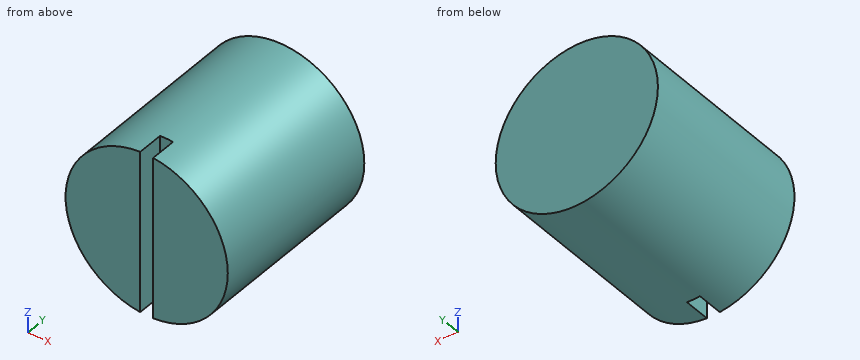
Autodesk Fusion 360 part; units mm, degrees
sketch "Sketch1" plane through (0, 0, 0) normal (0, 1, 0) x (1, 0, 0)
  circle A0 centre (0, 0) radius 5
  dimension "d1" = 10
extrude "Extrude1" add sketch "Sketch1" along normal blind 11
sketch "Sketch2" plane through (0, 0, 0) normal (1, 0, 0) x (0, 1, 0)
sketch "Sketch3" plane through (0, 0, 0) normal (0, 1, 0) x (1, 0, 0)
  circle A0 centre (0, 0) radius 5
  line L0 (-0.398, -4.9841) -> (-0.398, 4.9841)
  line L1 (0.398, 4.9841) -> (0.398, -4.9841)
  line L2 (-0.398, -4.9841) -> (-0.398, -5.1)
  line L3 (-0.398, -5.1) -> (0.4, -5.1)
  line L4 (0.4, -5.1) -> (0.398, -4.9841)
  line L5 (0.398, 4.9841) -> (0.398, 5.2684)
  line L6 (0.398, 5.2684) -> (-0.5, 5.2684)
  line L7 (-0.5, 5.2684) -> (-0.398, 4.9841)
extrude "Extrude2" cut sketch "Sketch3" along normal blind 1.6 contours A0 L0 L1 | A0 L5 L6 L7 | A0 L2 L3 L4
CAD build for the part. Positions are in the model's coordinates, mm. Give positions to 0.01 mm unless a question says otherwise; leave off trailing zeros. Order: outer loops, then holes, each group sorted by start corner. A loop starts at its lowest first (then second) coordinate and runs counter-clockwise, first axis right, second up. Notation, with made-up numbers: (-15, 13.5) - (4, 13.5) arc R4 ccw to (4, 17.5) - close; hole circle Ø11 at (37, -23.5). An arc over 180 degrees is marked (long way). Answer in a Markdown table with one row per item.
1. Saw through at A-A, the plane z = -3. Give the cut face in (x, y), plus the area to 3 significant figures.
Data:
| item | result |
|---|---|
| outline | (-4, 0) - (-0.4, 0) - (-0.4, 1.6) - (0.4, 1.6) - (0.4, 0) - (4, 0) - (4, 11) - (-4, 11) - close |
| area | 86.7 mm² |
2. Saw through at C-C, the plane x = 0. Give the cut face in (y, z).
Data:
| item | result |
|---|---|
| outline | (1.6, -5) - (11, -5) - (11, 5) - (1.6, 5) - close |
3. Saw through at D-D, the plane z = -4. Give the cut face in (x, y), plus the area to 3 significant figures.
Data:
| item | result |
|---|---|
| outline | (-3, 0) - (-0.4, 0) - (-0.4, 1.6) - (0.4, 1.6) - (0.4, 0) - (3, 0) - (3, 11) - (-3, 11) - close |
| area | 64.7 mm² |
4. Flat gauge pins, fed straight in: pin 1 (5 mm diameter, centred on y = 7, z = -3, fed in from -X); pin 2 (0.6 mm diameter, centred on x = 0, z = 1.5, fed in from -Y); pin 3 (1 mm diameter, centred on y = 2.5, z = -1.5, fed in from -X). Where does each tip first touch, or does it go through?
Data:
| item | result |
|---|---|
| pin 1 | stops at x = -4.97 |
| pin 2 | stops at y = 1.6 |
| pin 3 | stops at x = -4.9 |
5. Saw through at B-B, the plane y = 8. Give the cut face in (x, z).
Data:
| item | result |
|---|---|
| outline | circle Ø10 at (0, 0) |
6. Probe probe 1 along Y at (x, z) = (-0.25, -0.25); probe 2 along X at (y, z) = (6.75, -3.75); probe 3 along Z at (x, y) = (-3, 6.5). List the from-to ranges inside material, lowest first. Write a range as [from, to].
Data:
| item | result |
|---|---|
| probe 1 | y = [1.6, 11] |
| probe 2 | x = [-3.31, 3.31] |
| probe 3 | z = [-4, 4] |
